Study the drawing (mm; zero at the part's minimum x, y, z) and answer. A direction names the side the tool comes from. Give positions to 0.01 mm unless a question says otherwise; leave off trailing zeros. Loops run counter-clockwise (first coordinate to the right, second up) from the corner with the lowest first, then second, coordinate; pieces in that order, holes last. Notation, with made-up numbers: (-29.5, 83.25) - (-12.5, 83.25) arc R14 ccw to (-12.5, 95.25) - close; hole circle Ø7 at (12.5, 85.5). An arc over 180 degrees is marked (long way). Write item = value, one per line. Start each with the question number.
1) The mould has two halves that part along X. Classify the marked faces 3, 4 and 5: +X half, -X half, draft (parallel to the pull), parting line (faces both ways), or undercut.
2) The part is cut by section A-A on x = 16. Write down the section's boundary in (y, z), plus the area to 3 significant figures.
3) The part is cut by section C-C on z = 1.5. Write down the section's boundary in (x, y).
4) Which of the six approach directions +Z, -Z, +X, -X, +Y, -Y give full straight-line access (tool end or side, diameter ignored) to the marked faces 1 and 2?
5) Consider probe 1 along Z at (x, y) = (16, 1.05); probe 2 along Y at (x, z) = (10, 0.5); probe 3 along X at (y, z) = (13, 4.5). Determine where each line is inside the solid, lowest interval first.
6) The part is cut by section D-D on y = 2.75. Write down the section's boundary in (x, z), plus the area to 3 significant figures.
7) Flat-ended cylindrical pins translate along their axes: P1, Ø2, axis at y = 16, z = 3, coming from the +X side; P2, Ø0.8, axis at y = 19, z = 2, coming from the +X side; P3, Ø1.5, axis at x = 14.5, z = 4.5, coming from the +Y side; P4, Ø1.5, axis at y = 11, z = 2, coming from the +X side. Find the tip coordinate at first contact, or state that the pin passes through.
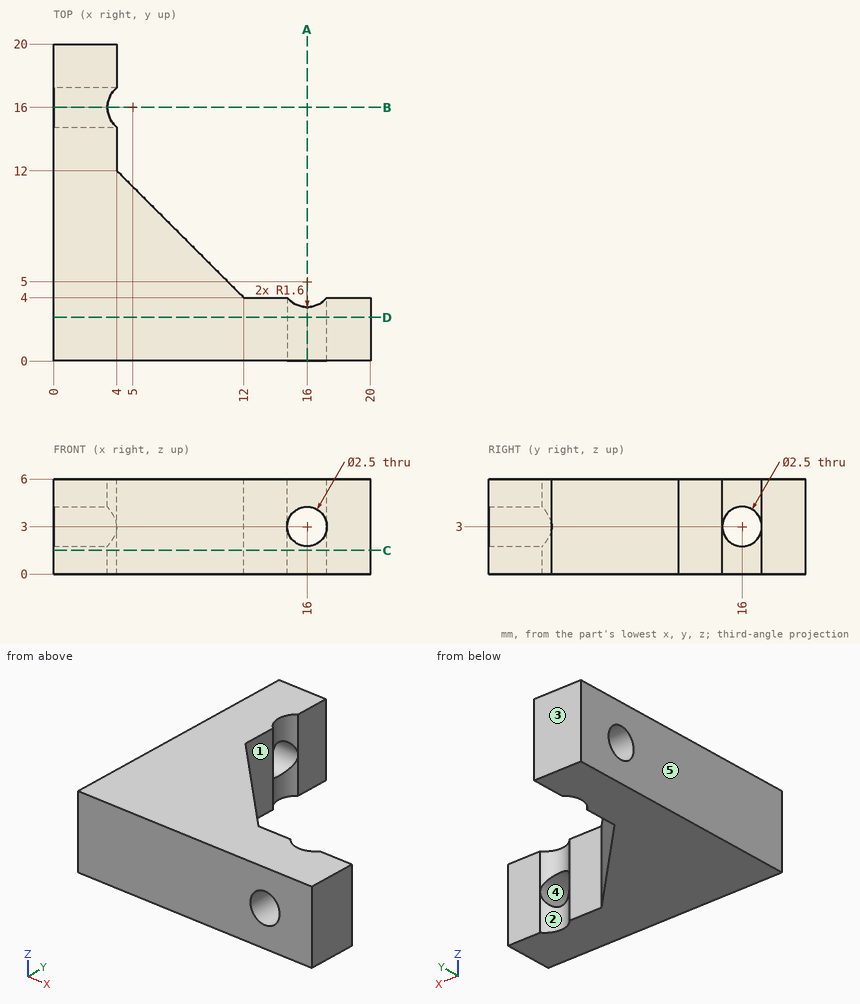
Answer below:
q1.face_3 = draft
q1.face_4 = undercut
q1.face_5 = -X half
q2.outline = (0, 0) - (3.4, 0) - (3.4, 1.75) - (0, 1.75) - close; (0, 4.25) - (3.4, 4.25) - (3.4, 6) - (0, 6) - close
q2.area = 11.9 mm2
q3.outline = (0, 0) - (20, 0) - (20, 4) - (17.25, 4) arc R1.6 cw to (14.75, 4) - (12, 4) - (4, 12) - (4, 14.75) arc R1.6 cw to (4, 17.25) - (4, 20) - (0, 20) - close
q4.face_1 = +Z, -Z, +X, +Y
q4.face_2 = +Z, -Z, +Y
q5.probe_1 = 0 to 1.75, 4.25 to 6
q5.probe_2 = 0 to 6
q5.probe_3 = 0 to 4
q6.outline = (0, 0) - (20, 0) - (20, 6) - (0, 6) - close; hole circle Ø2.5 at (16, 3)
q6.area = 115 mm2
q7.P1 = through
q7.P2 = 4
q7.P3 = 4
q7.P4 = 5.75
